```python
from build123d import *

# Parameters (mm, degrees)
F0_R     = 7
F1_DEPTH = 2


with BuildPart() as f1:
    # F0 (on Top) → F1 (new body)
    with BuildSketch(Plane.XY):
        with Locations((90, 12.5)):
            Circle(F0_R)
        with BuildLine():
            ThreePointArc((17, 12.5), (10, 19.5), (3, 12.5))
            ThreePointArc((3, 12.5), (10, 5.5), (17, 12.5))
        make_face()
        Polygon((0, 12.5), (0, 0), (100, 0), (100, 12.5), (100, 25), (0, 25), align=None)
        with BuildLine():
            ThreePointArc((17, 12.5), (10, 5.5), (3, 12.5))
            ThreePointArc((3, 12.5), (10, 19.5), (17, 12.5))
        make_face(mode=Mode.SUBTRACT)
        with Locations((90, 12.5)):
            Circle(F0_R, mode=Mode.SUBTRACT)
    extrude(amount=F1_DEPTH)


solid = f1.part
```
Work out the finished part from the listing and answer in its coordinate system (mm). Round coordinates to 2 decimals unless told otherwise and drop trailing zeros. Loops run counter-clockwise (first coordinate to the right, second up) from the corner with the lowest first, then second, coordinate; pieces in that order, holes last. Notation, with made-up numbers: M -26,75.25 L 21,75.25 A21 cw 21,82.25 Z; hole C 41,76.5 d2. An arc over 180 degrees is marked long. Use CSV: the item, a comma, the result in double quotes.
Q1. Section C-C, the plane z = 0.7 is taken. Determine the outline of the cut face in (x, y).
Determined:
outline,"M 0,0 L 100,0 L 100,25 L 0,25 Z; hole C 10,12.5 d14; hole C 90,12.5 d14"
Q2. Section D-D, the plane x = 9 is taken. Determine the outline of the cut face in (y, z).
Determined:
outline,"M 0,0 L 5.57,0 L 5.57,2 L 0,2 Z; M 19.43,0 L 25,0 L 25,2 L 19.43,2 Z"
Q3. Consider L1, parallel to Y at x = 10, z = 0.85; L2, parallel to X at y = 8.25, z = 1.2; L3, parallel to X at y = 8, z = 1.75. Determine where each line is inside the solid, lowest interval first.
Determined:
L1,"0 to 5.5, 19.5 to 25"
L2,"0 to 4.44, 15.56 to 84.44, 95.56 to 100"
L3,"0 to 4.64, 15.36 to 84.64, 95.36 to 100"
Q4. Section B-B, the plane y = 12.5 is taken. Determine the outline of the cut face in (x, z).
Determined:
outline,"M 0,0 L 3,0 L 3,2 L 0,2 Z; M 17,0 L 83,0 L 83,2 L 17,2 Z; M 97,0 L 100,0 L 100,2 L 97,2 Z"
Q5. Section A-A, the plane x = 90 is taken. Determine the outline of the cut face in (y, z), then the cut area to 3 significant figures.
Determined:
outline,"M 0,0 L 5.5,0 L 5.5,2 L 0,2 Z; M 19.5,0 L 25,0 L 25,2 L 19.5,2 Z"
area,"22.0 mm2"
